from build123d import *

# Parameters (mm, degrees)
BOSS_EXTRUDE1_DEPTH = 12.7
CUT_EXTRUDE1_START  = -13.521664
SKETCH2_R           = 9.525
CUT_EXTRUDE1_DEPTH  = 13.521664
SKETCH3_R           = 6.35
CUT_EXTRUDE2_DEPTH  = 77.878671194
FILLET3_START       = -1
FILLET3_DEPTH       = 26.4
CUT_EXTRUDE3_DEPTH  = 77.878671193
FILLET4_R           = 5.08


with BuildPart() as part:
    # Sketch1 → Boss-Extrude1 (new, symmetric)
    with BuildSketch(Plane.XY):
        Polygon((0, 0), (73.390309881, 0), (73.390309881, 15.548608999), (43.207324686, 25.4), (43.207324686, 6.35), (0, 6.35), align=None)
    extrude(amount=BOSS_EXTRUDE1_DEPTH, both=True)

    # Sketch2 → Cut-Extrude1 (cut)
    with BuildSketch(Plane(origin=(11.651871006, 35.699349465, 0), x_dir=(0.9506452030208671, -0.3102800315415328, 0), z_dir=(0.3102800315415327, 0.950645203020867, 0)).offset(CUT_EXTRUDE1_START)):
        with Locations(Location((49.068723147, 0, 0), (0, 0, 180))):
            Circle(SKETCH2_R)
    extrude(amount=CUT_EXTRUDE1_DEPTH, mode=Mode.SUBTRACT)

    # Sketch3 → Cut-Extrude2 (cut, through all)
    with BuildSketch(Plane(origin=(0, 6.35, 0), x_dir=(1, 0, 0), z_dir=(0, 1, 0))):
        with Locations(Location((21.603662343, 0, 0), (0, 0, 180))):
            Circle(SKETCH3_R)
    extrude(amount=-CUT_EXTRUDE2_DEPTH, mode=Mode.SUBTRACT)

    # Fillet3: read off the stored shape, not the designer's step
    # Fillet3 outline → Fillet3 (cut)
    with BuildSketch(Plane(origin=(0, 0, 0), x_dir=(1, 0, 0), z_dir=(0, 1, 0)).offset(FILLET3_START)):
        with BuildLine():
            ThreePointArc((60.690309881, 12.7), (69.670566002, 8.980256121), (73.390309881, 0))
            Line((73.390309881, 0), (73.390309881, 12.7))
            Line((73.390309881, 12.7), (60.690309881, 12.7))
        make_face()
        with BuildLine():
            ThreePointArc((73.390309881, 0), (69.670566002, -8.980256121), (60.690309881, -12.7))
            Line((60.690309881, -12.7), (73.390309881, -12.7))
            Line((73.390309881, -12.7), (73.390309881, 0))
        make_face()
    extrude(amount=FILLET3_DEPTH, mode=Mode.SUBTRACT)

    # Sketch4 → Cut-Extrude3 (cut, through all)
    with BuildSketch(Plane(origin=(0, 6.35, 0), x_dir=(1, 0, 0), z_dir=(0, 1, 0))):
        with BuildLine():
            Line((21.603662343, 12.7), (0, 12.7))
            Line((0, 12.7), (0, -12.7))
            Line((0, -12.7), (21.603662343, -12.7))
            ThreePointArc((21.603662343, -12.7), (8.903662343, 0), (21.603662343, 12.7))
        make_face()
    extrude(amount=-CUT_EXTRUDE3_DEPTH, mode=Mode.SUBTRACT)

    # Fillet4
    fillet4_edges = [part.edges().sort_by_distance(p)[0] for p in [
        (43.207324686, 6.35, 0),
    ]]
    fillet(fillet4_edges, radius=FILLET4_R)


solid = part.part
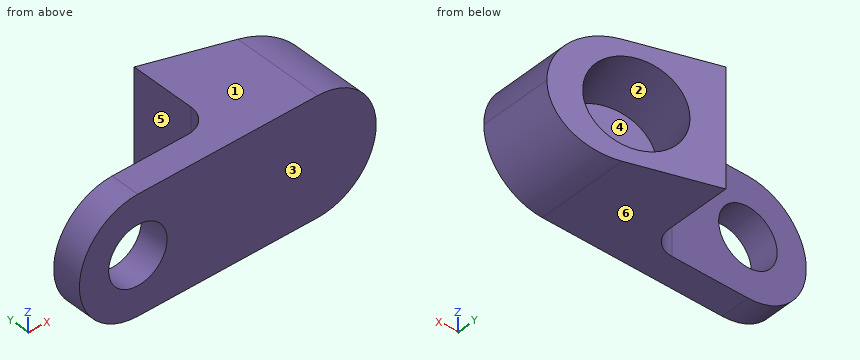
Verification items for the finished model (mm, model axes). Face numbers are marked on the shaded views. A direction names the side the tool comes from. Round coordinates to 2 decimals unless told otherwise and drop trailing zeros. Loops run counter-clockwise (first coordinate to the right, second up) from the corner with the lowest first, then second, coordinate; pieces in that order, holes last. Notation, with made-up numbers: (35, 7) - (64, 7) arc R13 ccw to (64, 31) - close; hole circle Ø4 at (-11.5, 50). An arc over 180 degrees is marked (long way). Answer in a Markdown table with one row per item. Add a question column.
Q1. Gauge pin test, flat ends, axial feed: pin 1 (2 mm diameter, centred on y = 21.5, z = -7, fed in from +X); pin 2 (1.5 mm diameter, centred on x = 19, z = -5, fed in from -Y); pin 3 (4 mm diameter, centred on y = 10, z = 8, fed in from -X); pin 4 (6 mm diameter, centred on x = 16, z = 6.5, fed in from +Y). Record the tip position at first contact, or that the pin passes through.
Q2. Material ranges on line 1 (Z direction, x = 18.5, y = 5.25); line 2 (Y direction, x = 34, z = 1.25); line 3 (Z direction, x = 59, y = 16), recorded low to high.
Q3. Tool access check on the marked faces 4, 5 and 6. Record the directions out of +Z, -Z, +X, -X, +Y, -Y that give a thin tool (end or side, any length) a straight path to the whole face; none if there is none.
Q4. Section check A-A on z = -1.25. Enter the section's corners in (x, y), plus the area to 3 significant figures.
Q5. Release check for a two-part mould opening along Z. For the marked faces 1, 2 and 3 record: pulls with the +Z half, pulls with the -Z half, needs draft (parallel to the pull), parting line crosses it, or undercut.
Q6. Section check B-B on x = 36. Enter the section's corners in (y, z).
Q7. Section check C-C on z = 4.5. Enter the section's corners in (x, y), plus the area to 3 significant figures.
Found:
| question | item | result |
|---|---|---|
| 1 | pin 1 | stops at x = 53.23 |
| 1 | pin 2 | stops at y = 0 |
| 1 | pin 3 | stops at x = 41.87 |
| 1 | pin 4 | stops at y = 6.35 |
| 2 | line 1 | z = -12.31 to -5.54, 5.54 to 12.31 |
| 2 | line 2 | y = 0 to 6.35 |
| 2 | line 3 | z = -12.7 to -9.3, 9.3 to 12.7 |
| 3 | face 4 | none |
| 3 | face 5 | +Z, -Z, -X, +Y |
| 3 | face 6 | -Z, +X, -X, +Y, -Y |
| 4 | outline | (8.97, 0) - (15.38, 0) - (15.38, 6.35) - (8.97, 6.35) - close; (27.83, 0) - (73.33, 0) - (73.33, 15.57) - (67.28, 17.54) - (63.08, 4.69) - (45.13, 10.55) - (49.32, 23.4) - (43.21, 25.4) - (43.21, 11.43) arc R5.08 cw to (38.13, 6.35) - (27.83, 6.35) - close |
| 4 | area | 506 mm² |
| 5 | face 1 | pulls with the +Z half |
| 5 | face 2 | undercut |
| 5 | face 3 | needs draft |
| 6 | outline | (0, -12.7) - (6.35, -12.7) - (6.35, 12.7) - (0, 12.7) - close |
| 7 | outline | (9.73, 0) - (17.12, 0) - (17.12, 6.35) - (9.73, 6.35) - close; (26.08, 0) - (72.57, 0) - (72.57, 15.82) - (66.28, 17.87) - (62.08, 5.02) - (46.12, 10.22) - (50.32, 23.08) - (43.21, 25.4) - (43.21, 11.43) arc R5.08 cw to (38.13, 6.35) - (26.08, 6.35) - close |
| 7 | area | 539 mm² |
